from build123d import *

# Parameters (mm, degrees)
F1_DEPTH = 63.5
F2_DEPTH = 25.4
F3_DEPTH = 7.9375
F0_W     = 25.4
F0_H     = 19.05
F5_R     = 6.35


with BuildPart() as f1:
    # F0 (on Front) → F1 (new body, symmetric)
    with BuildSketch(Plane.XZ):
        Polygon((-41.275, 9.525), (-41.275, -9.525), (41.275, -9.525), (41.275, 9.525), (22.225, 9.525), align=None)
    extrude(amount=F1_DEPTH, both=True)

    # F0 (on Front) → F2 (join, symmetric)
    with BuildSketch(Plane.XZ):
        with BuildLine():
            Line((22.225, 9.525), (41.275, 9.525))
            Line((41.275, 9.525), (41.275, 27.0002))
            ThreePointArc((41.275, 27.0002), (45.9246798487, 38.2255201513), (57.15, 42.8752))
            Line((57.15, 42.8752), (60.325, 42.8752))
            Line((60.325, 42.8752), (60.325, 61.9252))
            Line((60.325, 61.9252), (57.15, 61.9252))
            add(Edge.make_bspline(
                [(55.6525886726, 61.8930844368), (56.1562808572, 61.9065949604), (56.6554908346, 61.9172958156), (57.15, 61.9252)],
                knots=[109.9898733807, 109.9898733807, 109.9898733807, 109.9898733807, 111.5045361635, 111.5045361635, 111.5045361635, 111.5045361635], degree=3))
            ThreePointArc((55.6525886726, 61.8930844368), (31.9304370021, 51.1606897963), (22.225, 27.0002))
            Line((22.225, 27.0002), (22.225, 9.525))
        make_face()
    extrude(amount=F2_DEPTH, both=True)

    # F0 (on Front) → F3 (join, symmetric)
    with BuildSketch(Plane.XZ):
        with BuildLine():
            add(Edge.make_bspline(
                [(-41.275, 9.525), (-41.1359151521, 45.1149860549), (19.0761042936, 60.9119942548), (55.6525886726, 61.8930844368)],
                knots=[0, 0, 0, 0, 109.9898733807, 109.9898733807, 109.9898733807, 109.9898733807], degree=3))
            Line((-41.275, 9.525), (22.225, 9.525))
            Line((22.225, 9.525), (22.225, 27.0002))
            ThreePointArc((22.225, 27.0002), (31.9304370021, 51.1606897963), (55.6525886726, 61.8930844368))
        make_face()
    extrude(amount=F3_DEPTH, both=True)

    # F0 (on Front) → F4 (revolve)
    with BuildSketch(Plane.XZ):
        with Locations((73.025, 52.4002)):
            Rectangle(F0_W, F0_H)
    revolve(axis=Axis((60.325, 0, 52.3875), (0, 0, 1)))

    # F5
    f5_edges = [f1.edges().sort_by_distance(p)[0] for p in [
        (-41.275, 63.5, 0),
        (41.275, 63.5, 0),
        (-41.275, -63.5, 0),
        (41.275, -63.5, 0),
    ]]
    fillet(f5_edges, radius=F5_R)


solid = f1.part
The model under review builds one solid part; all positions refer to its coordinate system, in mm. A direction names the side the tool comes from. Round coordinates to 2 decimals unless told otherwise and drop trailing zeros. Order: outer loops, then holes, each group sorted by start corner. A loop starts at its lowest first (then second) coordinate and runs counter-clockwise, first axis right, second up. Notation, with made-up numbers: (76.25, 78.25) -> (98.25, 78.25) arc R13 cw to (98.25, 95.25) -> close; hole circle Ø10 at (-21.5, -27.5). An arc over 180 degrees is marked (long way). Write item = value, one per line. Start each with the question number.
Item 1: For line 1 along X through (y, z) = (5, -7) (3 decimals); line 2 along Z through (x, y) = (-1, 43) (3 decimals); line 3 along Y through (x, z) = (-10, 15.5), list the stretches that pass through material, from the lowest coordinate up.
Item 2: Consider section A-A on z = 2. Write out the cut boundary in (x, y) (3 decimals), plus the area to 3 significant figures.
Item 3: Consider section D-D on y = 43. Write out the cut boundary in (x, z) (3 decimals).
Item 4: Consider section B-B on x = 54. Write out the cut boundary in (y, z), plus the area to 3 significant figures.
Item 5: Clearance check with flat-ended pins moving along their axes: pin 1 Ø8 at (x, y) = (-5.5, 36.5) entering from +Z (3 decimals); pin 2 Ø8.5 at (y, z) = (-17.5, 20.5) entering from -X (3 decimals); pin 3 Ø11 at (y, z) = (24.5, 11) entering from +X (3 decimals). State where each tip first meets the part, or that it passes through.
Item 6: For faces 1 (the face through (68, 0, 42.875)), 2 (the face through (34.93, 0.51, 60.81)), 3 (the face through (37, 25.4, 36)), 4 (the face through (28.42, 16.55, 46.86)), 5 (the face through (22.225, -17, 18)), list the 3-axis set-ups (+Z, -Z, +X, -X, +Y, -Y) from which the entire face can be reached by the end or side of a thin tool; tool diameter is ignored.
Conclusion:
q1.line_1 = -41.275 to 41.275
q1.line_2 = -9.525 to 9.525
q1.line_3 = -7.94 to 7.94
q2.outline = (-41.275, -57.15) arc R6.35 ccw to (-34.925, -63.5) -> (34.925, -63.5) arc R6.35 ccw to (41.275, -57.15) -> (41.275, 57.15) arc R6.35 ccw to (34.925, 63.5) -> (-34.925, 63.5) arc R6.35 ccw to (-41.275, 57.15) -> close
q2.area = 10,400 mm2
q3.outline = (-41.275, -9.525) -> (41.275, -9.525) -> (41.275, 9.525) -> (-41.275, 9.525) -> close
q4.outline = (-25.4, 42.56) -> (25.4, 42.56) -> (25.4, 61.78) -> (24.6, 61.78) -> (24.6, 61.93) -> (-24.6, 61.93) -> (-24.6, 61.78) -> (-25.4, 61.78) -> close
q4.area = 984 mm2
q5.pin_1 = 9.525
q5.pin_2 = 22.225
q5.pin_3 = 41.275
q6.face_1 = -Z, +X, +Y, -Y
q6.face_2 = +Z, -X
q6.face_3 = +Z, +X, -X, +Y
q6.face_4 = +Z, -X, +Y
q6.face_5 = +Z, -X, -Y
